The listing builds one solid part. Answer for the finished solid, in the listing's coordinates (mm). Face numbers are marked on the shaded views. A direction names the side the tool comes from. Round coordinates to 2 decimals unless told otherwise and drop trailing zeros. Loops run counter-clockwise (first coordinate to the right, second up) from the corner with the lowest first, then second, coordinate; pieces in that order, holes last. Notation, with made-up numbers: (-26.75, -18) -> (22.25, -18) arc R7 cw to (22.25, -10) -> close; hole circle Ø11 at (13, 85). An arc over 180 degrees is marked (long way). Answer in a Markdown table with one row per item. Add a question column.
```python
from build123d import *

# Parameters (mm, degrees)
BOSS_EXTRUDE1_DEPTH                          = 2
CSK_FOR_M2_COUNTERSUNK_FLAT_HEAD_SCR_4_COUNT = 2
CSK_FOR_M2_COUNTERSUNK_FLAT_HEAD_SCR_4_PITCH = 10.825317547
CSK_FOR_M2_COUNTERSUNK_FLAT_HEAD_SCR_5_COUNT = 2
CSK_FOR_M2_COUNTERSUNK_FLAT_HEAD_SCR_5_PITCH = 10.825317547
BOSS_EXTRUDE2_START                          = -1
BOSS_EXTRUDE2_DEPTH                          = 1
FILLET1_R                                    = 7
CUT_EXTRUDE1_DEPTH                           = 1


# Read off the part's stored shape, not the designer's step: CSK for M2 Countersunk Flat Head Screw1
with BuildPart() as part:
    # Sketch1 → Boss-Extrude1 (new body)
    with BuildSketch(Plane(origin=(0, 0, 0), x_dir=(1, 0, 0), z_dir=(0, 1, 0))):
        with BuildLine():
            Line((4.5, 10.60416551), (4.5, 7.50416551))
            ThreePointArc((4.5, 7.50416551), (8.75, 0), (4.5, -7.50416551))
            Line((4.5, -7.50416551), (4.5, -10.60416551))
            ThreePointArc((4.5, -10.60416551), (0, -15.10416551), (-4.5, -10.60416551))
            Line((-4.5, -10.60416551), (-4.5, -7.50416551))
            ThreePointArc((-4.5, -7.50416551), (-8.75, 0), (-4.5, 7.50416551))
            Line((-4.5, 7.50416551), (-4.5, 10.60416551))
            ThreePointArc((-4.5, 10.60416551), (0, 15.10416551), (4.5, 10.60416551))
        make_face()
    extrude(amount=BOSS_EXTRUDE1_DEPTH)

    # CSK for M2 Countersunk Flat Head Scr 2 → CSK for M2 Countersunk Flat Head Screw1 (revolve, cut)
    with BuildSketch(Plane.XY.offset(10.60416551)):
        Polygon((0, 0), (1.1, 0), (1.1, 0.8), (2.3, 2), (0, 2), align=None)
    revolve(axis=Axis((0, 0, 10.60416551), (0, 1, 0)), mode=Mode.SUBTRACT)

    # CSK for M2 Countersunk Flat Head Scr 3 o → CSK for M2 Countersunk Flat Head Scr 3 (revolve, cut)
    with BuildSketch(Plane.XY.offset(-10.60416551)):
        Polygon((0, 0), (1.1, 0), (1.1, 0.8), (2.3, 2), (0, 2), align=None)
    revolve(axis=Axis((0, 0, -10.60416551), (0, 1, 0)), mode=Mode.SUBTRACT)

    # Sketch6 → CSK for M2 Countersunk Flat Head Screw2 (revolve, cut)
    with BuildSketch(Plane(origin=(6.25, 0, 0), x_dir=(0, 0, -1), z_dir=(1, 0, 0))):
        Polygon((0, 0), (0, 2), (1.1, 2), (1.1, 1.2), (2.3, 0), align=None)
    csk_for_m2_countersunk_flat_head_screw2 = revolve(axis=Axis((6.25, -6.35, 0), (0, 1, 0)), mode=Mode.SUBTRACT)

    # CSK for M2 Countersunk Flat Head Scr 4: CSK for M2 Countersunk Flat Head Screw2 ×2
    with Locations(*[Vector(-0.8660254037844379, 0, -0.5000000000000012) * (i * CSK_FOR_M2_COUNTERSUNK_FLAT_HEAD_SCR_4_PITCH) for i in range(1, CSK_FOR_M2_COUNTERSUNK_FLAT_HEAD_SCR_4_COUNT)]):
        add(csk_for_m2_countersunk_flat_head_screw2, mode=Mode.SUBTRACT)

    # CSK for M2 Countersunk Flat Head Scr 5: CSK for M2 Countersunk Flat Head Screw2 ×2
    with Locations(*[Vector(-0.8660254037844383, 0, 0.5000000000000008) * (i * CSK_FOR_M2_COUNTERSUNK_FLAT_HEAD_SCR_5_PITCH) for i in range(1, CSK_FOR_M2_COUNTERSUNK_FLAT_HEAD_SCR_5_COUNT)]):
        add(csk_for_m2_countersunk_flat_head_screw2, mode=Mode.SUBTRACT)

    # Sketch7 → Boss-Extrude2 (add)
    with BuildSketch(Plane(origin=(0, 2, 0), x_dir=(1, 0, 0), z_dir=(0, 1, 0)).offset(BOSS_EXTRUDE2_START)):
        with BuildLine():
            Line((4.5, 10.60416551), (10.5, 10.60416551))
            Line((10.5, 10.60416551), (10.5, -10.60416551))
            Line((10.5, -10.60416551), (4.5, -10.60416551))
            Line((4.5, -10.60416551), (4.5, -7.50416551))
            ThreePointArc((4.5, -7.50416551), (8.75, 0), (4.5, 7.50416551))
            Line((4.5, 7.50416551), (4.5, 10.60416551))
        make_face()
        with BuildLine():
            Line((-4.5, -7.50416551), (-4.5, -10.60416551))
            Line((-4.5, -10.60416551), (-10.5, -10.60416551))
            Line((-10.5, -10.60416551), (-10.5, 10.60416551))
            Line((-10.5, 10.60416551), (-4.5, 10.60416551))
            Line((-4.5, 10.60416551), (-4.5, 7.50416551))
            ThreePointArc((-4.5, 7.50416551), (-8.75, 0), (-4.5, -7.50416551))
        make_face()
    extrude(amount=BOSS_EXTRUDE2_DEPTH)

    # Fillet1
    # the kernel refuses this fillet: 7 mm, written as the material it takes off along each edge
    with BuildSketch(Plane(origin=(-10.5, -16.320508076, -10.60416551), x_dir=(1, 0, 0), z_dir=(0, 1, 0))) as fillet1_piece_1:
        with BuildLine():
            CenterArc((7, -6.92820323), FILLET1_R, 98.213210702, 81.786789298)
            Line((0, -6.92820323), (-0.14, -6.92820323))
            Line((-0.14, -6.92820323), (-0.14, 0))
            Line((-0.14, 0), (0, 0.14))
            ThreePointArc((0, 0.14), (3, 0.14), (5.98, 0.138564065))
            Line((5.98, 0.138564065), (6, 0))
        make_face()
    extrude(amount=35.641016151, mode=Mode.SUBTRACT)
    with BuildSketch(Plane(origin=(-10.5, -16.320508076, 10.60416551), x_dir=(1, 0, 0), z_dir=(0, 1, 0)), Plane(origin=(10.5, -16.320508076, -10.60416551), x_dir=(-1, 0, 0), z_dir=(0, 1, 0))) as fillet1_piece_2:
        with BuildLine():
            CenterArc((7, 6.92820323), FILLET1_R, 180, 81.786789298)
            Line((0, 6.92820323), (-0.14, 6.92820323))
            Line((-0.14, 6.92820323), (-0.14, 0))
            Line((-0.14, 0), (0, -0.14))
            ThreePointArc((0, -0.14), (3, -0.14), (5.98, -0.138564065))
            Line((5.98, -0.138564065), (6, 0))
        make_face()
    extrude(amount=35.641016151, mode=Mode.SUBTRACT)
    with BuildSketch(Plane(origin=(10.5, -16.320508076, 10.60416551), x_dir=(0, 0, -1), z_dir=(0, 1, 0))) as fillet1_piece_3:
        with BuildLine():
            CenterArc((6.92820323, 7), FILLET1_R, 188.213210702, 81.786789298)
            Line((0, 6), (-0.138564065, 5.98))
            ThreePointArc((-0.138564065, 5.98), (-0.14, 3), (-0.14, 0))
            Line((-0.14, 0), (0, -0.14))
            Line((0, -0.14), (6.92820323, -0.14))
            Line((6.92820323, -0.14), (6.92820323, 0))
        make_face()
    extrude(amount=35.641016151, mode=Mode.SUBTRACT)

    # Sketch8 → Cut-Extrude1 (cut)
    with BuildSketch(Plane.XZ):
        with BuildLine():
            Line((-4.5, -10.60416551), (-4.5, -7.50416551))
            ThreePointArc((-4.5, -7.50416551), (-8.75, 0), (-4.5, 7.50416551))
            Line((-4.5, 7.50416551), (-4.5, 10.60416551))
            ThreePointArc((-4.5, 10.60416551), (0, 15.10416551), (4.5, 10.60416551))
            Line((4.5, 10.60416551), (4.5, 7.50416551))
            ThreePointArc((4.5, 7.50416551), (8.75, 0), (4.5, -7.50416551))
            Line((4.5, -7.50416551), (4.5, -10.60416551))
            ThreePointArc((4.5, -10.60416551), (0, -15.10416551), (-4.5, -10.60416551))
        make_face()
        with BuildLine():
            Line((4.15, 7.3032527), (4.15, 10.60416551))
            ThreePointArc((4.15, 10.60416551), (0, 14.75416551), (-4.15, 10.60416551))
            Line((-4.15, 10.60416551), (-4.15, 7.3032527))
            ThreePointArc((-4.15, 7.3032527), (-8.4, 0), (-4.15, -7.3032527))
            Line((-4.15, -7.3032527), (-4.15, -10.60416551))
            ThreePointArc((-4.15, -10.60416551), (0, -14.75416551), (4.15, -10.60416551))
            Line((4.15, -10.60416551), (4.15, -7.3032527))
            ThreePointArc((4.15, -7.3032527), (8.4, 0), (4.15, 7.3032527))
        make_face(mode=Mode.SUBTRACT)
    extrude(amount=-CUT_EXTRUDE1_DEPTH, mode=Mode.SUBTRACT)


solid = part.part
```
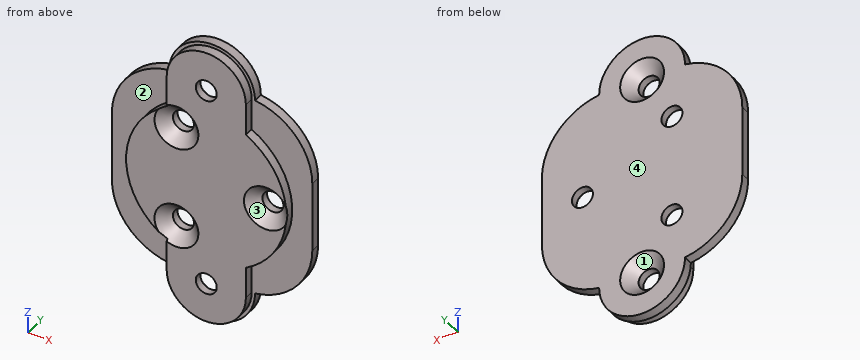
Item 1: The mould has two halves that part along Z. Classify the marked faces 3 and 4: +Z half, -Z half, draft (parallel to the pull), parting line (faces both ways), or undercut.
Item 2: For the marked faces 1 and 2, determine the directions among +Z, -Z, +X, -X, +Y, -Y from which every point of the face is accessible in a straight line to the end or side of a thin tool.
Item 3: Section A-A, the plane x = 0 is taken. Write down the section's boundary in (y, z).
Item 4: Consider L1, parallel to Z at x = 0, y = 0.6; L2, parallel to Z at x = -1.75, y = 1.65; L3, parallel to X at y = 0.35, z = -11. Determine where each line is inside the solid, lowest interval first. Write a range as from..to.
Item 5: Section C-C, the plane x = 6.25 is taken. Write down the section's boundary in (y, z).
Item 6: Section D-D, the plane x = -6.5 is taken. Write down the section's boundary in (y, z), and give its area (3 significant figures).
Item 7: Section B-B, the plane z = 0 is taken. Write down the section's boundary in (x, y).
Item 8: Flat-ended cylindrical pins translate along their axes: P1, Ø3, axis at x = 6.25, z = 0, coming from the -Y side; P2, Ø2.5, axis at x = -3.12, z = 5.41, coming from the -Y side; P3, Ø0.8, axis at y = 0.5, z = 8.5, coming from the +X side; P4, Ø1.3, axis at x = 0, z = 10.6, coming from the +Y side. Find the tip coordinate at first contact, or state that the pin passes through.
Here are the results:
| question | item | result |
|---|---|---|
| 1 | face 3 | undercut |
| 1 | face 4 | draft |
| 2 | face 1 | +Y |
| 2 | face 2 | -Y |
| 3 | outline | (0, -14.75) -> (1, -14.75) -> (1, -15.1) -> (2, -15.1) -> (2, -12.9) -> (0.8, -11.7) -> (0, -11.7) -> close; (0, -9.5) -> (0.8, -9.5) -> (2, -8.3) -> (2, 8.3) -> (0.8, 9.5) -> (0, 9.5) -> close; (0, 11.7) -> (0.8, 11.7) -> (2, 12.9) -> (2, 15.1) -> (1, 15.1) -> (1, 14.75) -> (0, 14.75) -> close |
| 4 | L1 | z = -14.75..-11.7, -9.5..9.5, 11.7..14.75 |
| 4 | L2 | z = -14.75..-11.46, -9.74..9.74, 11.46..14.75 |
| 4 | L3 | x = -4.13..-1.03, 1.03..4.13 |
| 5 | outline | (0, -5.61) -> (1, -5.61) -> (1, -10.11) -> (2, -10.11) -> (2, -1.1) -> (1.2, -1.1) -> (0, -2.3) -> close; (0, 2.3) -> (1.2, 1.1) -> (2, 1.1) -> (2, 10.11) -> (1, 10.11) -> (1, 5.61) -> (0, 5.61) -> close |
| 6 | outline | (0, -5.32) -> (1, -5.32) -> (1, -10) -> (2, -10) -> (2, 10) -> (1, 10) -> (1, 5.32) -> (0, 5.32) -> close |
| 6 | area | 30.6 mm² |
| 7 | outline | (-10.5, 1) -> (-8.4, 1) -> (-8.4, 0) -> (3.95, 0) -> (5.15, 1.2) -> (5.15, 2) -> (-10.5, 2) -> close; (7.35, 1.2) -> (8.4, 0.15) -> (8.4, 1) -> (10.5, 1) -> (10.5, 2) -> (7.35, 2) -> close |
| 8 | P1 | stops at y = 0.8 |
| 8 | P2 | stops at y = 1.04 |
| 8 | P3 | stops at x = 4.15 |
| 8 | P4 | passes through |
